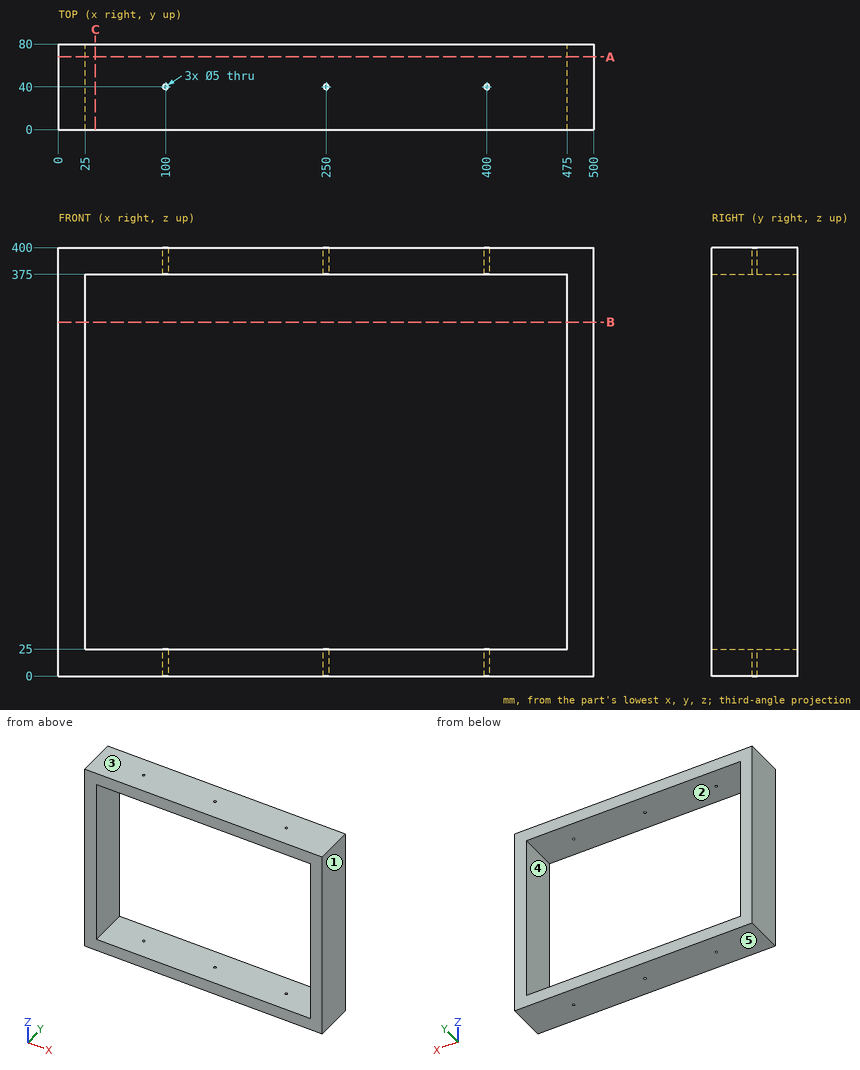
Answer from the drawing. Dimensions are ordinates in mm from the lowest x, y and z of the part. A direction names the side the tool comes from. Coordinates: 2 decimals unless noted, no trailing zeros. Order: outer loops, then holes, each group sorted by start corner. A loop starts at its lowest first (then second) coordinate and runs counter-clockwise, first axis right, second up. Notation, with made-up numbers: (-24.75, -26.5) - (-0.75, -26.5) arc R9 ccw to (-0.75, -9.5) - close; hole circle Ø4 at (20, 65.25). An arc over 180 degrees is marked (long way). Put each result on its own line as item: value. Start each with the question number.
1) Find section B-B (z = 330.5). Give the vertices of the cut face in (x, y).
2) Find section C-C (x = 34.5). Give the vertices of the cut face in (y, z).
3) For the marked faces 1 and 2, determine the directions among +Z, -Z, +X, -X, +Y, -Y from which every point of the face is accessible in a straight line to the end or side of a thin tool.
4) Find the intervals of material crossed by line 1 (Z direction, x = 334, y = 52); line 2 (X direction, y = 36, z = 115.5); line 3 (Y direction, x = 400, z = 393), in increasing order. Write a range as from..to.
5) Find section A-A (y = 68). Give the vertices of the cut face in (x, z), plus the area to 3 significant figures.
6) For a pull along Z with two mould halves and no side action, classify the marked faces 3, 4 and 5 as released by +Z, released by -Z, zero draft, split by the parting line, or undercut.
Results list:
1. outline: (0, 0) - (25, 0) - (25, 80) - (0, 80) - close; (475, 0) - (500, 0) - (500, 80) - (475, 80) - close
2. outline: (0, 0) - (80, 0) - (80, 25) - (0, 25) - close; (0, 375) - (80, 375) - (80, 400) - (0, 400) - close
3. face 1: +Z, -Z, +X, +Y, -Y
3. face 2: +Y, -Y
4. line 1: z = 0..25, 375..400
4. line 2: x = 0..25, 475..500
4. line 3: y = 0..37.5, 42.5..80
5. outline: (0, 0) - (500, 0) - (500, 400) - (0, 400) - close; hole (25, 25) - (475, 25) - (475, 375) - (25, 375) - close
5. area: 42,500 mm^2
6. face 3: released by +Z
6. face 4: undercut
6. face 5: released by -Z
